```python
from build123d import *

# Parameters (mm, degrees)
F0_R     = 8.5
F0_R_2   = 5
F1_DEPTH = 6.35


with BuildPart() as f1:
    # F0 (on Front) → F1 (new body)
    with BuildSketch(Plane.XZ):
        with BuildLine():
            Line((-31.4690486828, -40), (0, -40))
            Line((0, -40), (31.4690486828, -40))
            ThreePointArc((31.4690486828, -40), (45.7816462008, -22.233800758), (50.895, 0))
            ThreePointArc((50.895, 0), (-22.233800758, 45.7816462008), (-31.4690486828, -40))
        make_face()
        with BuildLine():
            ThreePointArc((0, -40), (-28.2842712475, 28.2842712475), (40, 0))
            ThreePointArc((40, 0), (28.2842712475, -28.2842712475), (0, -40))
        make_face(mode=Mode.SUBTRACT)
        with BuildLine():
            ThreePointArc((0, -40), (28.2842712475, -28.2842712475), (40, 0))
            ThreePointArc((40, 0), (-28.2842712475, 28.2842712475), (0, -40))
        make_face()
        with Locations((0, -20)):
            Circle(F0_R, mode=Mode.SUBTRACT)
        Circle(F0_R_2, mode=Mode.SUBTRACT)
    extrude(amount=F1_DEPTH)


solid = f1.part
```
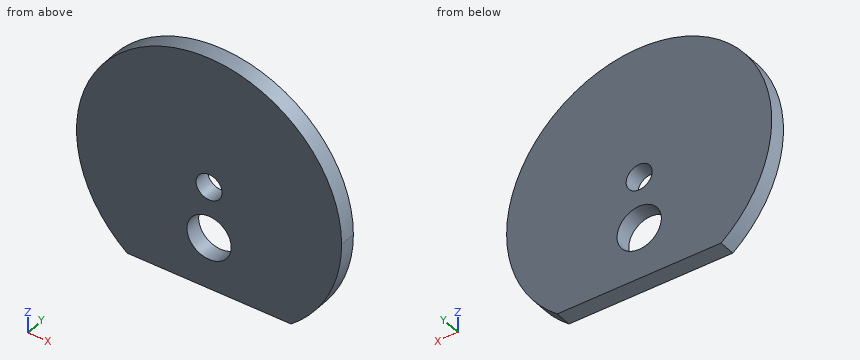
Can you work these out from the model? Positions are in its coordinate system, mm. Round coordinates to 2 decimals unless told otherwise and drop trailing zeros. Loops run counter-clockwise (first coordinate to the right, second up) from the corner with the lowest first, then second, coordinate; pieces in that order, holes last. Notation, with made-up numbers: M 8.25,82.25 L 32.25,82.25 A23 cw 32.25,110.25 Z; hole C 35.25,83 d10. An arc over 180 degrees is marked long. Answer in a Markdown table with one row per item.
1. I'm going to push a flat-ended pin straight in: pin 1 Ø1.5 at (y, z) = (-1, 5.5) entering from -X. Where does the tip first touch, or does it pass through?
Established:
| item | result |
|---|---|
| pin 1 | x = -50.67 |
2. If we section it at C-C, the plane y = -2.25: Please give me the cut outline in (x, z) (3 decimals), plus the area to 3 significant figures.
Established:
| item | result |
|---|---|
| outline | M -31.469,-40 L 31.469,-40 A50.895 ccw long Z; hole C 0,-20 d17; hole C 0,0 d10 |
| area | 7,360 mm² |
3. If we section it at A-A, the plane z = -26: Please give me the cut outline in (x, y).
Established:
| item | result |
|---|---|
| outline | M -43.75,-6.35 L -6.02,-6.35 L -6.02,0 L -43.75,0 Z; M 6.02,-6.35 L 43.75,-6.35 L 43.75,0 L 6.02,0 Z |
4. Please list where these lines run through material, in increasing order: line 1 (Z direction, x = 0, y = -2.75) (3 decimals); line 2 (X direction, y = -4, z = -22); line 3 (Z direction, x = -6, y = -6). Write a range as from..to.
Established:
| item | result |
|---|---|
| line 1 | -40..-28.5, -11.5..-5, 5..50.895 |
| line 2 | -45.89..-8.26, 8.26..45.89 |
| line 3 | -40..-26.02, -13.98..50.54 |
5. If we section it at D-D, the plane x = 35: Please give me the cut outline in (y, z).
Established:
| item | result |
|---|---|
| outline | M -6.35,-36.95 L 0,-36.95 L 0,36.95 L -6.35,36.95 Z |
6. If we section it at B-B, the plane x = 0: Please give me the cut outline in (y, z) (3 decimals), plus the area to 3 significant figures.
Established:
| item | result |
|---|---|
| outline | M -6.35,-40 L 0,-40 L 0,-28.5 L -6.35,-28.5 Z; M -6.35,-11.5 L 0,-11.5 L 0,-5 L -6.35,-5 Z; M -6.35,5 L 0,5 L 0,50.895 L -6.35,50.895 Z |
| area | 406 mm² |
